Autodesk Inventor part; units mm, degrees
ref_plane "Start Plane" through (0, 0, -16.764) normal (0, 0, 1) x (1, 0, 0)
ref_plane "End Plane" through (0, 0, 86.764) normal (0, 0, 1) x (1, 0, 0)
ref_plane "Work Plane4" through (0, -16.764, -16.764) normal (0, 0.7071, -0.7071) x (1, 0, 0)
ref_plane "Start Plane" through (0, 0, -16.764) normal (0, 0, 1) x (1, 0, 0)
ref_plane "End Plane" through (0, 0, 86.764) normal (0, 0, 1) x (1, 0, 0)
sketch "Sketch" plane through (0, 0, 0) normal (0, 0, 1) x (1, 0, 0)
  circle A0 centre (0, 0) radius 12.2174
  circle A1 centre (0, 0) radius 16.764
  dimension "d0" = 33.528
  dimension "d1" = 4.5466
extrude "Body" add sketch "Sketch" along normal up to surface (103.528 mm away) from surface at -16.764
sketch "Sketch3" plane through (0, 0, 0) normal (0, 0, 1) x (1, 0, 0)
  line L0 (0, 0) -> (10, 0)
ref_plane "Work Plane3" through (0, 0, 0) normal (0, -1, 0) x (1, 0, 0)
ref_plane "Work Plane4" through (0, -16.764, -16.764) normal (0, 0.7071, -0.7071) x (1, 0, 0)
split "Split1" plane through (0, -16.764, -16.764) removes the side toward (0, 0.7071, -0.7071)
ref_plane "Work Plane5" through (0, -16.764, 86.764) normal (0, 0.7071, 0.7071) x (1, 0, 0)
split "Split2" plane through (0, -16.764, 86.764) removes the side toward (0, 0.7071, 0.7071)
sketch "Sketch4" plane through (0, 0, 0) normal (0, -1, 0) x (1, 0, 0)
  line L0 (-2, -16.764) -> (12, -16.764)
  line L1 (-2, 86.764) -> (12, 86.764)
  dimension "d7" = 103.528
equation "\"d0\" = G_H"
equation "\"d1\" = G_T"
equation "\"d2\" = G_L"
equation "\"G_H\" = 33.528"
equation "\"G_T\" = 4.5466"
equation "\"G_L\" = d7"
equation "\"G_OFFSET_START\" = 16.764"
equation "\"G_OFFSET_END\" = 16.764"
equation "\"d4\" = -G_OFFSET_START"
equation "\"d5\" = G_OFFSET_END + B_L"
equation "\"B_L\" = 70"
properties part number "ANSI - 1 x 0.179 - 4.076" material "Steel, Mild"
Could you check a few things on this model? Use its own coordinates, in mm. Give positions to 0.01 mm unless a question says otherwise; leave off trailing zeros. Order: outer loops, then holes, each group sorted by start corner. A loop starts at its lowest first (then second) coordinate and runs counter-clockwise, first axis right, second up. Notation, with made-up numbers: (38.25, 33.5) - (76.25, 33.5) arc R13 ccw to (76.25, 37.5) - close; hole circle Ø1 at (65.25, 60.5). An arc over 180 degrees is marked (long way). Return JSON: item names as keys, results as strings. Group by question number.
Q1. Suppose I cut it at D-D, the plane z = 68. Please give me the cut outline in (x, y).
Q2. Thinking about a two-plate mould opening in Y: for faces 1 (the face through (-2.18, -16.62, 34.28)), 2 (the face through (-1.59, -12.113, 34.338)), 3 (the face through (12.34, 1.16, 68.84)), which applies, pulls with the +Y half, pulls with the -Y half, needs draft (parallel to the pull), parting line crosses it, or undercut?
Q3. Will these pins go through, and if not, where does the flat tip stop? pin 1 Ø2 at (y, z) = (-13, 71) entering from -X; pin 2 Ø6 at (x, z) = (-9.5, 63) entering from -Y; pin 3 Ø2 at (y, z) = (11, 46) entering from -X.
Q4. Suppose I cut it at B-B, the plane x = 0. Please give me the cut outline in (y, z).
Q5. Suppose I cut it at C-C, the plane z = 50. Please give me the cut outline in (x, y), and give its area (3 significant figures).
Q6. Please list where these lines run through material, in increasing order: line 1 along Y through (x, z) = (0, 32); line 2 along X through (y, z) = (-9, 17). Write a range as [from, to].
Resolved:
{
 "1": {"outline": "(-16.64, 2) arc R16.76 ccw (long way) to (16.64, 2) - (12.05, 2) arc R12.22 cw (long way) to (-12.05, 2) - close"},
 "2": {"face 1": "parting line crosses it", "face 2": "undercut", "face 3": "pulls with the +Y half"},
 "3": {"pin 1": "stops at x = -11.71", "pin 2": "stops at y = -15.45", "pin 3": "stops at x = -13.45"},
 "4": {"outline": "(-16.76, -16.76) - (-12.22, -12.22) - (-12.22, 82.22) - (-16.76, 86.76) - close; (12.22, 12.22) - (16.76, 16.76) - (16.76, 53.24) - (12.22, 57.78) - close"},
 "5": {"outline": "circle Ø33.53 at (0, 0); hole circle Ø24.43 at (0, 0)", "area": "414 mm2"},
 "6": {"line 1": "y = [-16.76, -12.22], [12.22, 16.76]", "line 2": "x = [-14.14, -8.26], [8.26, 14.14]"}
}
